Work out the finished part from the listing and answer in its coordinate system (mm). Face numbers are marked on the shaded views. A direction names the side the tool comes from. Coordinates: 2 decimals unless noted, no trailing zeros. Order: outer loops, then holes, each group sorted by start corner. A loop starts at its lowest first (then second) coordinate and runs counter-clockwise, first axis right, second up. Notation, with made-up numbers: M 63,68.5 L 115,68.5 A31 cw 115,101.5 Z; hole C 5.5,82 d4. An arc over 180 degrees is marked long. Use a Markdown table: item, result. Add a question column.
from build123d import *

# Parameters (mm, degrees)
F0_W     = 320.675
F0_H     = 101.6
F1_DEPTH = 7.9375
F3_D     = 12.7
F5_DEPTH = 368.3
F7_DEPTH = 265.1135
F8_W     = 327.025
F8_H     = 50.8
F9_DEPTH = 7.9375


with BuildPart() as f1:
    # F0 (on Front) → F1 (new body)
    with BuildSketch(Plane.XZ):
        with Locations((0, -50.8)):
            Rectangle(F0_W, F0_H)
    extrude(amount=F1_DEPTH)

    # F3 (through all)
    with Locations(Plane.XZ.offset(7.9375)):
        with Locations((-128.5875, -19.05), (128.5875, -19.05), (128.5875, -82.55), (-128.5875, -82.55)):
            Hole(F3_D / 2)

    # F4 (on face) → F5 (join)
    with BuildSketch(Plane.XZ.offset(7.9375)):
        Polygon((-96.8375, 0), (-160.3375, 0), (-160.3375, -7.9375), (-104.775, -7.9375), (-104.775, -101.6), (-96.8375, -101.6), align=None)
        Polygon((160.3375, 0), (96.8375, 0), (96.8375, -101.6), (104.775, -101.6), (104.775, -7.9375), (160.3375, -7.9375), align=None)
    extrude(amount=F5_DEPTH)

    # F6 (on face) → F7 (cut, through all)
    with BuildSketch(Plane(origin=(-104.775, 0, 0), x_dir=(0, -1, 0), z_dir=(-1, 0, 0))):
        Polygon((376.2375, -101.6), (376.2375, -7.9375), (249.2375, -101.6), align=None)
    extrude(amount=-F7_DEPTH, mode=Mode.SUBTRACT)

    # F8 (on face) → F9 (join)
    with BuildSketch(Plane.XY):
        with Locations((0, -122.2375)):
            Rectangle(F8_W, F8_H)
        with Locations((0, -350.8375)):
            Rectangle(F8_W, F8_H)
    extrude(amount=F9_DEPTH)


solid = f1.part
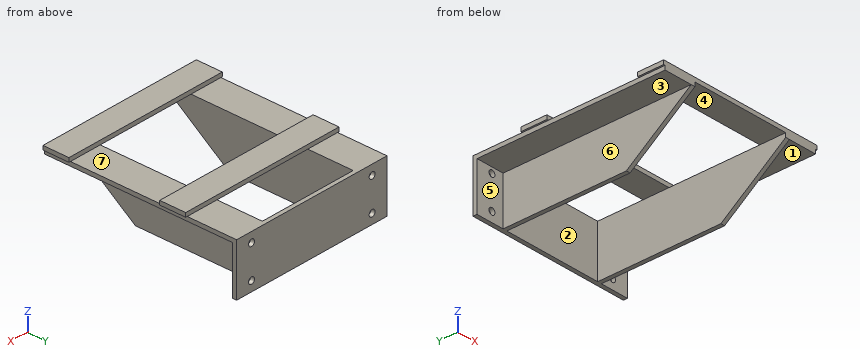
(1) Given P1, Ø3.5, axis at x = 162, y = -121, coming from the -Z side; P2, Ø8.5, axis at x = 2, z = 5.5, coming from the +Y side; P3, Ø2.5, axis at x = -162, y = -130, coming from the -Z side, each flat-ended and moving along its own axis, determine where each tip first touches the part or whether it passes through.
(2) A cutting plane is placed at D-D on z = -37. Write down the section's boundary in (x, y) (1 decimal).
(3) A cutting plane is placed at A-A on y = -192.5. Write down the section's boundary in (x, z) (1 decimal).
(4) A cutting plane is placed at B-B on x = -28. Write down the section's boundary in (y, z), plus the area to 3 significant figures.
(5) A cutting plane is placed at C-C on z = -19.05. Write down the section's boundary in (x, y) (1 decimal).
(6) Straight lines are drawn through the part: line 1 (X direction, y = -5, z = -82); line 2 (X direction, y = -169, z = -88) (1 decimal); line 3 (Y direction, x = -149.5, z = -41.5). For each, find the intervals that lie inside material, in ascending order.
(7) The mould has two halves that part along Y. Classify the marked faces 5, 6 and 7: pulls with the +Y half, pulls with the -Y half, needs draft (parallel to the pull), parting line crosses it, or undercut.
(8) Which of the six approach directions +Z, -Z, +X, -X, +Y, -Y give full straight-line access (tool end or side, diameter ignored) to the marked faces 1, 2, 3 and 4?
From the geometry:
| question | item | result |
|---|---|---|
| 1 | P1 | stops at z = -7.94 |
| 1 | P2 | stops at y = -96.84 |
| 1 | P3 | stops at z = 0 |
| 2 | outline | M -160.3,-7.9 L -104.8,-7.9 L -104.8,-336.8 L -96.8,-336.8 L -96.8,-7.9 L 96.8,-7.9 L 96.8,-336.8 L 104.8,-336.8 L 104.8,-7.9 L 160.3,-7.9 L 160.3,0 L -160.3,0 Z |
| 3 | outline | M -160.3,-7.9 L -104.8,-7.9 L -104.8,-101.6 L -96.8,-101.6 L -96.8,0 L -160.3,0 Z; M 96.8,-101.6 L 104.8,-101.6 L 104.8,-7.9 L 160.3,-7.9 L 160.3,0 L 96.8,0 Z |
| 4 | outline | M -376.24,0 L -325.44,0 L -325.44,7.94 L -376.24,7.94 Z; M -147.64,0 L -96.84,0 L -96.84,7.94 L -147.64,7.94 Z; M -7.94,-101.6 L 0,-101.6 L 0,0 L -7.94,0 Z |
| 4 | area | 1,610 mm2 |
| 5 | outline | M -160.3,-7.9 L -134.9,-7.9 L -134.9,0 L -160.3,0 Z; M -122.2,-7.9 L -104.8,-7.9 L -104.8,-361.2 L -96.8,-361.2 L -96.8,-7.9 L 96.8,-7.9 L 96.8,-361.2 L 104.8,-361.2 L 104.8,-7.9 L 122.2,-7.9 L 122.2,0 L -122.2,0 Z; M 134.9,-7.9 L 160.3,-7.9 L 160.3,0 L 134.9,0 Z |
| 6 | line 1 | x = -160.34 to -134.91, -122.26 to 122.26, 134.91 to 160.34 |
| 6 | line 2 | x = -104.8 to -96.8, 96.8 to 104.8 |
| 6 | line 3 | y = -7.94 to 0 |
| 7 | face 5 | pulls with the -Y half |
| 7 | face 6 | needs draft |
| 7 | face 7 | undercut |
| 8 | face 1 | -Z, +X, -Y |
| 8 | face 2 | +Z, -Z, -Y |
| 8 | face 3 | -Z, -X, -Y |
| 8 | face 4 | -Z, -Y |
